```python
from build123d import *

# Parameters (mm, degrees)
CROQUIS3_W              = 10
CROQUIS3_H              = 10
CROQUIS3_R              = 1.75
SALIENTE_EXTRUIR1_DEPTH = 50
SALIENTE_EXTRUIR2_DEPTH = 5
CROQUIS9_W              = 10
CROQUIS9_H              = 10
CROQUIS9_R              = 1.75
SALIENTE_EXTRUIR4_DEPTH = 15
CHAFL_N1_SIZE           = 1


with BuildPart() as part:
    # Croquis3 → Saliente-Extruir1 (new body)
    with BuildSketch(Plane(origin=(0, 0, 0), x_dir=(1, 0, 0), z_dir=(0, 1, 0))):
        with Locations((30, 0)):
            Rectangle(CROQUIS3_W, CROQUIS3_H)
        with Locations(Location((30, 0, 0), (0, 0, 270))):
            Circle(CROQUIS3_R, mode=Mode.SUBTRACT)
    extrude(amount=SALIENTE_EXTRUIR1_DEPTH)

    # Croquis4 → Saliente-Extruir2 (add)
    with BuildSketch(Plane.XY):
        Polygon((0, 0), (0, 4.066369454), (25, 42.555355948), (25, 35.154579698), (2.165818783, 0), align=None)
    extrude(amount=SALIENTE_EXTRUIR2_DEPTH)

    # Simetría1: part across plane


with BuildPart() as part_1:
    add(part.part)
    add(part.part.mirror(Plane.ZX))

    # Croquis9 → Saliente-Extruir4 (add)
    with BuildSketch(Plane.XZ.offset(50)):
        with Locations((30, -10)):
            Rectangle(CROQUIS9_W, CROQUIS9_H)
        with Locations(Location((30, -10, 0), (0, 0, 270))):
            Circle(CROQUIS9_R, mode=Mode.SUBTRACT)
    extrude(amount=-SALIENTE_EXTRUIR4_DEPTH)

    # Chaflán1
    chafl_n1_edges = [part_1.edges().sort_by_distance(p)[0] for p in [
        (30, -35, -15),
    ]]
    chamfer(chafl_n1_edges, length=CHAFL_N1_SIZE)

    # Simetría2: part across plane


with BuildPart() as part_2:
    add(part_1.part)
    add(part_1.part.mirror(Plane(origin=(0, 0, 0), x_dir=(0, 0, 1), z_dir=(1, 0, 0))))


solid = part_2.part
```
Could you check a few things on this model? Use its own coordinates, in mm. A direction names the side the tool comes from. Coordinates: 2 decimals unless noted, no trailing zeros. Write each loop counter-clockwise with the first axis right and the second up, starting at its lowest first coordinate (ties: lowest second). Pieces come first, ordered by that corner, then holes. Notation, with made-up numbers: (11.5, 53.25) -> (66.5, 53.25) arc R5 cw to (66.5, 59.25) -> close; hole circle Ø7 at (30.5, 56). An arc over 180 degrees is marked (long way). One line per question, with ' | ' between items. Start each with the question number.
1. If we section it at A-A (x = 30): Please give me the cut outline in (y, z).
2. If we section it at D-D (x = -9.5): Please give me the cut outline in (y, z).
3. Please list where these lines run through material, in increasing order: line 1 along Z through (x, y) = (-30, -39); line 2 along X through (y, z) = (16.5, -4.75); line 3 along Z through (x, y) = (-30, -23).
4. Will these pins go through, and if not, where does the flat tip stop? P1, Ø8, axis at x = -29.5, y = 8.5, coming from the -Z side; P2, Ø2.5, axis at x = 28, z = -8, coming from the +Y side; P3, Ø12, axis at x = 3, y = 17.5, coming from the -Z side.
5. For faces 4 (the face through (13.74, 17.82, 2.46)), 5 (the face through (31, -35, -8)), 6 (the face through (-12.3, -23, 2.5)), which set-ups out of +Z, -Z, +X, -X, +Y, -Y let a thin tool reach every point of the face, with its end or its side?
6. If we section it at B-B (z = -7.25): Please give me the cut outline in (x, y), and give its area (3 significant figures).
7. Thinking about a two-plate mould opening in Z: for faces 1 (the face through (30.526, -42.605, -11.669)), 2 (the face through (-30, 8, -5)), 3 (the face through (-13.74, 17.82, 2.46)), which applies, pulls with the +Z half, pulls with the -Z half, needs draft (parallel to the pull), parting line crosses it, or undercut?
8. If we section it at C-C (y = -37): Please give me the cut outline in (x, z), and give its area (3 significant figures).
Return value:
1) outline: (-50, -15) -> (-36, -15) -> (-35, -14) -> (-35, -11.75) -> (-50, -11.75) -> close; (-50, -8.25) -> (-35, -8.25) -> (-35, -5) -> (50, -5) -> (50, -1.75) -> (-50, -1.75) -> close; (-50, 1.75) -> (50, 1.75) -> (50, 5) -> (-50, 5) -> close
2) outline: (-18.69, 0) -> (-11.29, 0) -> (-11.29, 5) -> (-18.69, 5) -> close; (11.29, 0) -> (18.69, 0) -> (18.69, 5) -> (11.29, 5) -> close
3) line 1: z = -15 to -11.75, -8.25 to -1.75, 1.75 to 5 | line 2: x = -35 to -25, 25 to 35 | line 3: z = -5 to -1.75, 1.75 to 5
4) P1: stops at z = -5 | P2: stops at y = -35 | P3: stops at z = 0
5) face 4: +Z, -Z | face 5: -Z, +X, -X, +Y | face 6: +Z, -Z, -Y
6) outline: (-35, -50) -> (-25, -50) -> (-25, -35) -> (-35, -35) -> close; (25, -50) -> (35, -50) -> (35, -35) -> (25, -35) -> close | area: 300 mm²
7) face 1: undercut | face 2: pulls with the -Z half | face 3: needs draft
8) outline: (-35, -15) -> (-25, -15) -> (-25, 0) -> (-21.39, 0) -> (-21.39, 5) -> (-35, 5) -> close; (21.39, 0) -> (25, 0) -> (25, -15) -> (35, -15) -> (35, 5) -> (21.39, 5) -> close; hole circle Ø3.5 at (-30, -10); hole circle Ø3.5 at (-30, 0); hole circle Ø3.5 at (30, -10); hole circle Ø3.5 at (30, 0) | area: 398 mm²
